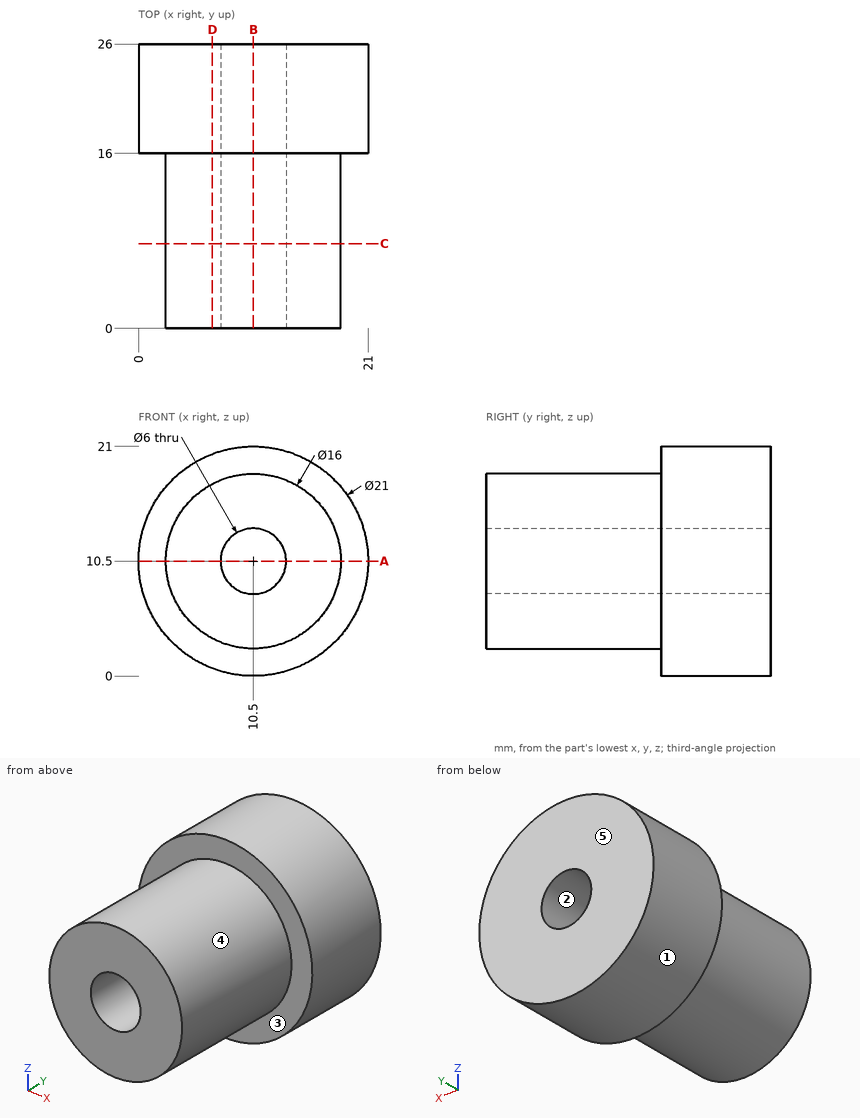
Check sheet for the drawn part. Datum: minimum x, y, z corner. Units: mm. A direction names the side the tool comes from. Round coordinates to 2 decimals unless told otherwise and drop trailing zeros. Order: outer loops, then holes, each group sorted by start corner. A loop starts at its lowest first (then second) coordinate and runs counter-clockwise, first axis right, second up.
1) Scan lines: line 1 (X direction, y = 11, z = 10.5); line 2 (Y direction, x = 13.5, z = 19); line 3 (X direction, y = 21.25, z = 10.5). Record each from-to range of solid material in increasing order.
2) Section check B-B (x = 10.5). Record the boundary of the cut face in (y, z), and give its area (3 significant figures).
3) Mould release check, pull along Z, two halves, no side actions. Record for the marked faces 1, 2 and 3: +Z half, -Z half, draft (parallel to the pull), parting line (faces both ways), or undercut.
4) Section check D-D (x = 6.75). Record the boundary of the cut face in (y, z), and give its area (3 significant figures).
5) Tool access check on the marked faces 4 and 5. Record the directions out of +Z, -Z, +X, -X, +Y, -Y that give a thin tool (end or side, any length) a straight path to the whole face; none if there is none.
6) Go/stop test with flat-tipped pins: pin 1 Ø12 at (x, y) = (2.5, 11.5) entering from +Z; pin 2 Ø4 at (x, y) = (3, 16) entering from -Z; pin 3 Ø12 at (y, z) = (4.5, 8.5) entering from -X. Record where each tip stops, or that it passes through.
7) Section check A-A (z = 10.5). Record the boundary of the cut face in (x, y), and give its area (3 significant figures).
8) Section check C-C (y = 7.75). Record the boundary of the cut face in (x, z).
Result:
1. line 1: x = 2.5 to 7.5, 13.5 to 18.5
1. line 2: y = 16 to 26
1. line 3: x = 0 to 7.5, 13.5 to 21
2. outline: (0, 2.5) - (16, 2.5) - (16, 0) - (26, 0) - (26, 7.5) - (0, 7.5) - close; (0, 13.5) - (26, 13.5) - (26, 21) - (16, 21) - (16, 18.5) - (0, 18.5) - close
2. area: 310 mm2
3. face 1: parting line
3. face 2: undercut
3. face 3: draft
4. outline: (0, 3.43) - (16, 3.43) - (16, 0.69) - (26, 0.69) - (26, 20.31) - (16, 20.31) - (16, 17.57) - (0, 17.57) - close
4. area: 422 mm2
5. face 4: -Y
5. face 5: +Z, -Z, +X, -X, +Y
6. pin 1: stops at z = 20.2
6. pin 2: stops at z = 1.56
6. pin 3: stops at x = 2.5
7. outline: (0, 16) - (2.5, 16) - (2.5, 0) - (7.5, 0) - (7.5, 26) - (0, 26) - close; (13.5, 0) - (18.5, 0) - (18.5, 16) - (21, 16) - (21, 26) - (13.5, 26) - close
7. area: 310 mm2
8. outline: circle Ø16 at (10.5, 10.5); hole circle Ø6 at (10.5, 10.5)
